For this review, take the finished solid that the model builds, in its own axes (mm). A direction names the side the tool comes from. Coordinates: 2 decimals unless noted, no trailing zeros. Write each loop counter-clockwise with the first axis right and the second up, starting at its lowest first coordinate (ties: lowest second). Pieces come first, ordered by that corner, then holes. Notation, with made-up numbers: M 87,-25.75 L 142,-25.75 A6 cw 142,-16.75 Z; hole C 50,52.25 d5. An arc over 180 degrees is marked long. One line per question, with ' | ' between items.
from build123d import *

# Parameters (mm, degrees)
SKETCH_2_R      = 1.75
EXTRUDE_1_DEPTH = 1
EXTRUDE_2_DEPTH = 2.5


with BuildPart() as part:
    # Эскиз2 → Бобышка-Вытянуть1 (new body)
    with BuildSketch(Plane(origin=(0, 0, 0), x_dir=(1, 0, 0), z_dir=(0, 1, 0))):
        Polygon((-35.5, 28), (-35.5, -28), (-34, -28), (-34, -34), (-28, -34), (-28, -35.5), (28, -35.5), (28, -34), (34, -34), (34, -28), (35.5, -28), (35.5, 28), (34, 28), (34, 34), (28, 34), (28, 35.5), (-28, 35.5), (-28, 34), (-34, 34), (-34, 28), align=None)
        with Locations((28, -28)):
            Circle(SKETCH_2_R, mode=Mode.SUBTRACT)
        with Locations((-28, -28)):
            Circle(SKETCH_2_R, mode=Mode.SUBTRACT)
        with Locations((-28, 28)):
            Circle(SKETCH_2_R, mode=Mode.SUBTRACT)
        with BuildLine():
            Line((20, 19), (20, 6.525504327))
            ThreePointArc((20, 6.525504327), (20.292893219, 5.818397545), (21, 5.525504327))
            Line((21, 5.525504327), (23, 5.525504327))
            ThreePointArc((23, 5.525504327), (23.707106781, 5.232611108), (24, 4.525504327))
            Line((24, 4.525504327), (24, -3.474495673))
            ThreePointArc((24, -3.474495673), (23.707106781, -4.181602455), (23, -4.474495673))
            Line((23, -4.474495673), (21, -4.474495673))
            ThreePointArc((21, -4.474495673), (20.292893219, -4.767388892), (20, -5.474495673))
            Line((20, -5.474495673), (20, -19))
            ThreePointArc((20, -19), (19.707106781, -19.707106781), (19, -20))
            Line((19, -20), (-19, -20))
            ThreePointArc((-19, -20), (-19.707106781, -19.707106781), (-20, -19))
            Line((-20, -19), (-20, -5.474495673))
            ThreePointArc((-20, -5.474495673), (-20.292893219, -4.767388892), (-21, -4.474495673))
            Line((-21, -4.474495673), (-23, -4.474495673))
            ThreePointArc((-23, -4.474495673), (-23.707106781, -4.181602455), (-24, -3.474495673))
            Line((-24, -3.474495673), (-24, 4.418145483))
            ThreePointArc((-24, 4.418145483), (-23.707106781, 5.125252264), (-23, 5.418145483))
            Line((-23, 5.418145483), (-21, 5.418145483))
            ThreePointArc((-21, 5.418145483), (-20.292893219, 5.711038701), (-20, 6.418145483))
            Line((-20, 6.418145483), (-20, 19))
            ThreePointArc((-20, 19), (-19.707106781, 19.707106781), (-19, 20))
            Line((-19, 20), (19, 20))
            ThreePointArc((19, 20), (19.707106781, 19.707106781), (20, 19))
        make_face(mode=Mode.SUBTRACT)
        with BuildLine():
            ThreePointArc((-32.375246916, -5.328874762), (-32.81067753, 0.113838264), (-32.337490331, 5.553398796))
            ThreePointArc((-32.337490331, 5.553398796), (-30.509920838, 9.7779661), (-29.531671369, 5.280188077))
            ThreePointArc((-29.531671369, 5.280188077), (-29.999989805, -0.024733046), (-29.522924885, -5.328874762))
            ThreePointArc((-29.522924885, -5.328874762), (-30.949085901, -6.755035778), (-32.375246916, -5.328874762))
        make_face(mode=Mode.SUBTRACT)
        with BuildLine():
            ThreePointArc((5.553398796, 32.337490331), (9.7779661, 30.509920838), (5.280188077, 29.531671369))
            ThreePointArc((5.280188077, 29.531671369), (-0.024733046, 29.999989805), (-5.328874762, 29.522924885))
            ThreePointArc((-5.328874762, 29.522924885), (-6.755035778, 30.949085901), (-5.328874762, 32.375246916))
            ThreePointArc((-5.328874762, 32.375246916), (0.113838264, 32.81067753), (5.553398796, 32.337490331))
        make_face(mode=Mode.SUBTRACT)
        with BuildLine():
            ThreePointArc((32.337490331, -5.553398796), (30.509920838, -9.7779661), (29.531671369, -5.280188077))
            ThreePointArc((29.531671369, -5.280188077), (29.999989805, 0.024733046), (29.522924885, 5.328874762))
            ThreePointArc((29.522924885, 5.328874762), (30.949085901, 6.755035778), (32.375246916, 5.328874762))
            ThreePointArc((32.375246916, 5.328874762), (32.81067753, -0.113838264), (32.337490331, -5.553398796))
        make_face(mode=Mode.SUBTRACT)
        with BuildLine():
            ThreePointArc((-5.553398796, -32.337490331), (-9.7779661, -30.509920838), (-5.280188077, -29.531671369))
            ThreePointArc((-5.280188077, -29.531671369), (0.024733046, -29.999989805), (5.328874762, -29.522924885))
            ThreePointArc((5.328874762, -29.522924885), (6.755035778, -30.949085901), (5.328874762, -32.375246916))
            ThreePointArc((5.328874762, -32.375246916), (-0.113838264, -32.81067753), (-5.553398796, -32.337490331))
        make_face(mode=Mode.SUBTRACT)
    extrude(amount=EXTRUDE_1_DEPTH)

    # Эскиз3 → Бобышка-Вытянуть2 (add, symmetric)
    with BuildSketch(Plane.XY):
        Polygon((-25, 0), (-24, 0), (-24, -17), (-20.953427174, -17), (-20.953427174, -18), (-25, -18), align=None)
        Polygon((25, 0), (25, -18), (20.953427174, -18), (20.953427174, -17), (24, -17), (24, 0), align=None)
    extrude(amount=EXTRUDE_2_DEPTH, both=True)


solid = part.part
1) To check wall thickness, follow line 1 along X through (y, z) = (-12.25, 1); line 2 along Y through (x, z) = (-20.5, 9). State the ranges of each line that lie inside material, in increasing order. Write a range as [from, to].
Responses:
line 1: [-25, -24], [24, 25] | line 2: [0, 1]
2) Insertion check: pin 1 Ø2.5 at (y, z) = (-6, -1) entering from +X; pin 2 Ø10 at (x, z) = (-7.5, -16) entering from -Y; pin 3 Ø4.5 at (x, y) = (23, -10.5) entering from +Z; pin 4 Ø5.5 at (x, z) = (28, 28) entering from +Y. Each pin has a flat end and moves straight along its axis. Give the tip position at first contact, or say it passes through.
Responses:
pin 1: x = 25 | pin 2: y = 0 | pin 3: z = 2.5 | pin 4: y = 1
3) We need section C-C on x = -31. State the section outline as (y, z) points, then the cut area to 3 significant figures.
Responses:
outline: M 0,-34 L 1,-34 L 1,-9.78 L 0,-9.78 Z; M 0,6.75 L 1,6.75 L 1,34 L 0,34 Z | area: 51.5 mm^2
4) The part is to be moulded in two halves that separate along Z. For faces 1 (the cylindrical face through (-30.595, 0.493, -9.785)), 2 (the flat face through (22, -17, 0)), 3 (the flat face through (-24.3, -9.6, 2.5)), say which applies: +Z half, -Z half, draft (parallel to the pull), parting line (faces both ways), or undercut.
Responses:
face 1: undercut | face 2: draft | face 3: +Z half
5) We need section B-B on x = 0. State the section outline as (y, z) points, then the cut area to 3 significant figures.
Responses:
outline: M 0,-35.5 L 1,-35.5 L 1,-32.81 L 0,-32.81 Z; M 0,-30 L 1,-30 L 1,-20 L 0,-20 Z; M 0,20 L 1,20 L 1,30 L 0,30 Z; M 0,32.81 L 1,32.81 L 1,35.5 L 0,35.5 Z | area: 25.4 mm^2
6) Machinability: for faces 4 (the flat face through (-25, -9, 0)), 5 (the flat face through (-24.3, -9.6, -2.5)), 6 (the flat face through (25, -9, 0)), which of the approach directions +Z, -Z, +X, -X, +Y, -Y give a long, thin tool a straight path to every point of the face, cutting with its end or side? Answer none if there is none.
Responses:
face 4: +Z, -Z, -X, -Y | face 5: -Z, +X, -X, -Y | face 6: +Z, -Z, +X, -Y
7) We need section A-A on y = -9.5. State the section outline as (x, z) points.
Responses:
outline: M -25,-2.5 L -24,-2.5 L -24,2.5 L -25,2.5 Z; M 24,-2.5 L 25,-2.5 L 25,2.5 L 24,2.5 Z
